Geometry check sheet. Reference: the model listing, model coordinates, mm. Round coordinates to 2 decimals unless told otherwise and drop trailing zeros. Order: outer loops, then holes, each group sorted by start corner. A loop starts at its lowest first (then second) coordinate and runs counter-clockwise, first axis right, second up.
(1) Sectioned sample at C-C (x = -15.5). Record the boundary of the cut face in (y, z) (3 decimals), plus the area to 3 significant figures.
(2) Material ranges on line 1 along X through (y, z) = (0.55, -46.85); line 2 along X through (y, z) = (0.1, 14.5) (3 decimals); line 3 along X through (y, z) = (1.3, -7), recorded low to high.
(3) Release check for a two-part mould opening along Z. For faces 1 (the face through (1, 0, -1)), 2 (the face through (-42.54, 1.25, 80.74)), 3 (the face through (28.375, 1.252, -48.358)), 4 (the face through (-3.98, 1.25, 15.92)) record: +Z half, -Z half, draft (parallel to the pull), parting line (faces both ways), or undercut.
(4) Go/stop test with flat-tipped pins: pin 1 (2 mm diameter, centred on x = 29, z = -69.85, fed in from +Y); pin 2 (4 mm diameter, centred on x = 15.875, z = -34.15, fed in from +Y). Record where each tip stops, or that it passes through.
(5) Sectioned sample at A-A (z = -15.1). Record the boundary of the cut face in (x, y), plus the area to 3 significant figures.
(6) Sectioned sample at B-B (z = -34.15). Record the boundary of the cut face in (x, y), plus the area to 3 significant figures.
(7) Sectioned sample at D-D (y = 1.25). Give the number of separate pieces and of enclosed holes in the cut face, plus the area to 3 significant figures.
from build123d import *

# Parameters (mm, degrees)
SKETCH1_R             = 1.4732
BOSS_EXTRUDE1_DEPTH   = 2.54
F_4_CLEARANCE_HOLE1_D = 3.2639
CUT_EXTRUDE1_REACH    = 95.791
SKETCH4_W             = 25.4
SKETCH4_H             = 63.5
SKETCH4_H_2           = 41.91


with BuildPart() as part:
    # Sketch1 → Boss-Extrude1 (new body)
    with BuildSketch(Plane(origin=(0, 0, 0), x_dir=(1, 0, 0), z_dir=(0, 1, 0))):
        with BuildLine():
            ThreePointArc((-44.45, 76.2), (-42.590128061, 80.690128061), (-38.1, 82.55))
            Line((-38.1, 82.55), (38.1, 82.55))
            ThreePointArc((38.1, 82.55), (42.590128061, 80.690128061), (44.45, 76.2))
            Line((44.45, 76.2), (44.45, -76.2))
            ThreePointArc((44.45, -76.2), (42.590128061, -80.690128061), (38.1, -82.55))
            Line((38.1, -82.55), (-38.1, -82.55))
            ThreePointArc((-38.1, -82.55), (-42.590128061, -80.690128061), (-44.45, -76.2))
            Line((-44.45, -76.2), (-44.45, 76.2))
        make_face()
        with Locations(Location((31.75, 19.05, 0), (0, 0, 270))):
            Circle(SKETCH1_R, mode=Mode.SUBTRACT)
        with Locations(Location((-31.75, 19.05, 0), (0, 0, 270))):
            Circle(SKETCH1_R, mode=Mode.SUBTRACT)
    extrude(amount=BOSS_EXTRUDE1_DEPTH)

    # #4 Clearance Hole1 (through all)
    with Locations(Plane(origin=(-29, 2.54, -69.85), x_dir=(0, 0, 1), z_dir=(0, 1, 0))):
        with Locations((0, 0), (0, 58), (23, 58), (23, 0), (39.8275, 5.53), (39.8275, 24.53), (87.3275, 24.53), (87.3275, 5.53), (35.7, 44.875), (54.75, 44.875)):
            Hole(F_4_CLEARANCE_HOLE1_D / 2)

    # Sketch4 → Cut-Extrude1 (cut, up to next)
    with BuildSketch(Plane(origin=(0, 2.54, 0), x_dir=(1, 0, 0), z_dir=(0, 1, 0)), mode=Mode.PRIVATE) as cut_extrude1_sk1:
        with Locations((22.225, -25.4)):
            Rectangle(SKETCH4_W, SKETCH4_H)
    cut_extrude1_tool1 = extrude(cut_extrude1_sk1.sketch, amount=-CUT_EXTRUDE1_REACH, mode=Mode.PRIVATE) & part.part
    # Sketch4 → Cut-Extrude1 (cut, up to next)
    with BuildSketch(Plane(origin=(0, 2.54, 0), x_dir=(1, 0, 0), z_dir=(0, 1, 0)), mode=Mode.PRIVATE) as cut_extrude1_sk2:
        with Locations((-13.97, 6.21)):
            Rectangle(SKETCH4_W, SKETCH4_H_2)
    cut_extrude1_tool2 = extrude(cut_extrude1_sk2.sketch, amount=-CUT_EXTRUDE1_REACH, mode=Mode.PRIVATE) & part.part
    add(cut_extrude1_tool1.solids().sort_by_distance((22.225, 2.54, 25.4))[0], mode=Mode.SUBTRACT)
    add(cut_extrude1_tool2.solids().sort_by_distance((-13.97, 2.54, -6.21))[0], mode=Mode.SUBTRACT)


solid = part.part
Answer below:
1. outline: (0, -82.55) - (2.54, -82.55) - (2.54, -27.165) - (0, -27.165) - close; (0, 14.745) - (2.54, 14.745) - (2.54, 82.55) - (0, 82.55) - close
1. area: 313 mm2
2. line 1: x = -44.45 to -30.63, -27.37 to 27.37, 30.63 to 44.45
2. line 2: x = -44.45 to -26.67, -1.27 to 9.525, 34.925 to 44.45
2. line 3: x = -44.45 to -26.67, -1.27 to 44.45
3. face 1: draft
3. face 2: +Z half
3. face 3: undercut
3. face 4: undercut
4. pin 1: passes through
4. pin 2: stops at y = 2.54
5. outline: (-44.45, 0) - (-26.67, 0) - (-26.67, 2.54) - (-44.45, 2.54) - close; (-1.27, 0) - (14.24, 0) - (14.24, 2.54) - (-1.27, 2.54) - close; (17.51, 0) - (44.45, 0) - (44.45, 2.54) - (17.51, 2.54) - close
5. area: 153 mm2
6. outline: (-44.45, 0) - (14.24, 0) - (14.24, 2.54) - (-44.45, 2.54) - close; (17.51, 0) - (44.45, 0) - (44.45, 2.54) - (17.51, 2.54) - close
6. area: 218 mm2
7. separate pieces: 1
7. enclosed holes: 14
7. area: 11,900 mm2
